```python
from build123d import *

# Parameters (mm, degrees)
EXTRUDE_1_DEPTH = 63.2
EXTRUDE_START   = -31.6
EXTRUDE_4_DEPTH = 15


with BuildPart() as part:
    # 草图1 → 拉伸-薄壁1 (new body)
    with BuildSketch(Plane.XY):
        with BuildLine():
            Line((-14, 5.385164807), (-14, -5.385164807))
            ThreePointArc((-14, -5.385164807), (15, 0), (-14, 5.385164807))
        make_face()
        with BuildLine():
            Line((-4, 3), (-4, -3))
            ThreePointArc((-4, -3), (5, 0), (-4, 3))
        make_face(mode=Mode.SUBTRACT)
    extrude(amount=EXTRUDE_1_DEPTH)

    # 草图9 → 拉伸-薄壁4 (add, symmetric)
    with BuildSketch(Plane.XY.offset(63.2).offset(EXTRUDE_START)):
        Polygon((-14, -5.385164807), (4.341640192, -37.153817513), (8.671767211, -34.653817513), (-9.669872981, -2.885164807), align=None)
    extrude(amount=EXTRUDE_4_DEPTH, both=True)


solid = part.part
```
CAD build for the part. Positions are in the model's coordinates, mm. A direction names the side the tool comes from. Round coordinates to 2 decimals unless told otherwise and drop trailing zeros. Write each loop counter-clockwise with the first axis right and the second up, starting at its lowest first coordinate (ties: lowest second). Pieces come first, ordered by that corner, then holes.
Item 1: Band-saw the part on C-C on x = 0. Write the cut outline in (y, z).
Filled in:
outline: (-29.63, 16.6) - (-19.63, 16.6) - (-19.63, 46.6) - (-29.63, 46.6) - close; (-15, 0) - (-5, 0) - (-5, 63.2) - (-15, 63.2) - close; (5, 0) - (15, 0) - (15, 63.2) - (5, 63.2) - close
Item 2: Band-saw the part on A-A on y = 0. Write the cut outline in (x, z).
Filled in:
outline: (-14, 0) - (-4, 0) - (-4, 63.2) - (-14, 63.2) - close; (5, 0) - (15, 0) - (15, 63.2) - (5, 63.2) - close
Item 3: Band-saw the part on B-B on z = 32. Write the cut outline in (x, y), then the cut area to 3 significant figures.
Filled in:
outline: (-14, -5.39) arc R15 ccw to (-11.66, -9.43) - (4.34, -37.15) - (8.67, -34.65) - (-2.83, -14.73) arc R15 ccw (long way) to (-14, 5.39) - close; hole (-4, -3) arc R5 ccw (long way) to (-4, 3) - close
area: 756 mm2
Item 4: Tool access for faces 4 (the flat face through (-4, 0, 31)), 5 (the flat face through (-6, 0, 0)): list every direction of +Z, -Z, +X, -X, +Y, -Y with a clear straight run to the whole face (end or side of a thin tool).
Filled in:
face 4: +Z, -Z
face 5: -Z, +X, -X, +Y, -Y
Item 5: Mould opens along Y. For faces 1 (the flat face through (-6, 0, 63.2)), 2 (the cylindrical face through (5, 0, 31)), 3 (the flat face through (6.48, -35.92, 31.81)) say: released by +Y, released by -Y, zero draft, split by the parting line, or undercut.
Filled in:
face 1: zero draft
face 2: undercut
face 3: released by -Y
Item 6: Band-saw the part on D-D on x = -7. Write the cut outline in (y, z), then the cut area to 3 significant figures.
Filled in:
outline: (-17.51, 16.6) - (-13.27, 16.6) - (-13.27, 0) - (13.27, 0) - (13.27, 63.2) - (-13.27, 63.2) - (-13.27, 46.6) - (-17.51, 46.6) - close
area: 1,800 mm2
Item 7: Drill centre lines: L1, parallel to X at y = 0, z = 43; L2, parallel to Y at x = 2.5, z = 23.5; L3, parallel to Y at x = 0, z = 31. Where is each one in solid material? Low to high.
Filled in:
L1: x = -14 to -4, 5 to 15
L2: y = -33.96 to -23.96, -14.79 to -4.33, 4.33 to 14.79
L3: y = -29.63 to -19.63, -15 to -5, 5 to 15
Item 8: Drop flat-ended pins along their axis: pin 1 Ø6 at (x, z) = (11.5, 18.5) entering from -Y; pin 2 Ø1.5 at (x, z) = (-11, 45.5) entering from -Y; pin 3 Ø5 at (y, z) = (-13.5, 13.5) entering from -X. Give the stop position or say it passes through.
Filled in:
pin 1: stops at y = -34.75
pin 2: stops at y = -11.88
pin 3: stops at x = -10.2
